Part print with two shaded views. Sizes in mm from the minimum x, y, z corner. Round coordinates to 2 decimals unless told otherwise and drop trailing zeros. Loops run counter-clockwise (first coordinate to the right, second up) from the corner with the lowest first, then second, coordinate; pieces in that order, holes last. Notation, with made-up numbers: (-33, 30) -> (23, 30) arc R26 ccw to (23, 67) -> close; hole circle Ø9 at (-14, 21). An arc over 180 degrees is marked (long way). Use a Markdown table: item, result. Add a question column.
Item 1: Probe line 1 (X direction, y = 74, z = 0.9); line 2 (Y direction, x = 23, z = 0.55). List the from-to ranges inside material, lowest first. Write a range as [from, to].
Item 2: Cut at B-B, the plane x = 7. List the corners of the cut face in (y, z), plus the area to 3 significant figures.
Item 3: Cut at A-A, the plane y = 22. List the corners of the cut face in (x, z), plus the area to 3 significant figures.
Item 4: Cut at C-C, the plane z = 1.1. State how many separate pieces and enclosed holes the cut face has, plus the area to 4 significant figures.
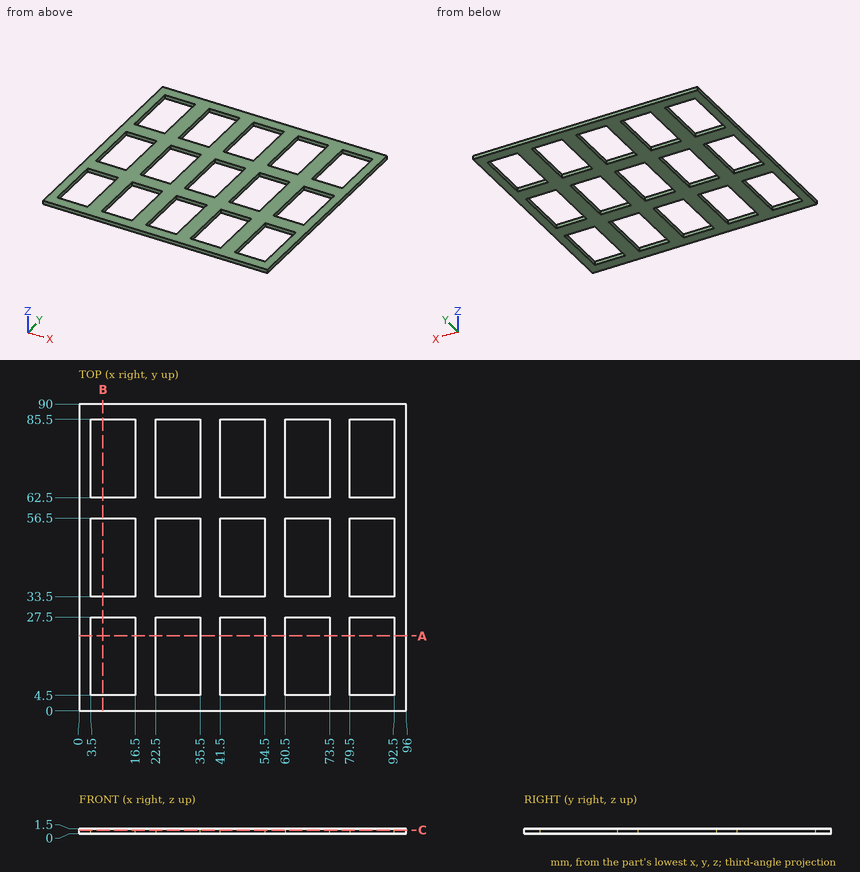
A:
| question | item | result |
|---|---|---|
| 1 | line 1 | x = [0, 3.5], [16.5, 22.5], [35.5, 41.5], [54.5, 60.5], [73.5, 79.5], [92.5, 96] |
| 1 | line 2 | y = [0, 4.5], [27.5, 33.5], [56.5, 62.5], [85.5, 90] |
| 2 | outline | (0, 0) -> (4.5, 0) -> (4.5, 1.5) -> (0, 1.5) -> close; (27.5, 0) -> (33.5, 0) -> (33.5, 1.5) -> (27.5, 1.5) -> close; (56.5, 0) -> (62.5, 0) -> (62.5, 1.5) -> (56.5, 1.5) -> close; (85.5, 0) -> (90, 0) -> (90, 1.5) -> (85.5, 1.5) -> close |
| 2 | area | 31.5 mm^2 |
| 3 | outline | (0, 0) -> (3.5, 0) -> (3.5, 1.5) -> (0, 1.5) -> close; (16.5, 0) -> (22.5, 0) -> (22.5, 1.5) -> (16.5, 1.5) -> close; (35.5, 0) -> (41.5, 0) -> (41.5, 1.5) -> (35.5, 1.5) -> close; (54.5, 0) -> (60.5, 0) -> (60.5, 1.5) -> (54.5, 1.5) -> close; (73.5, 0) -> (79.5, 0) -> (79.5, 1.5) -> (73.5, 1.5) -> close; (92.5, 0) -> (96, 0) -> (96, 1.5) -> (92.5, 1.5) -> close |
| 3 | area | 46.5 mm^2 |
| 4 | separate pieces | 1 |
| 4 | enclosed holes | 15 |
| 4 | area | 4,155 mm^2 |
